from build123d import *

# Parameters (mm, degrees)
BOSS_EXTRUDE10_DEPTH = 2
SKETCH14_R           = 3
SKETCH14_R_2         = 5.05
BOSS_EXTRUDE11_DEPTH = 8


with BuildPart() as part:
    # Sketch13 → Boss-Extrude10 (new body)
    with BuildSketch(Plane(origin=(-28.225984218, 0, 0), x_dir=(-1, 0, 0), z_dir=(0, -1, 0))):
        with BuildLine():
            Line((-40.725984218, 11), (-15.725984218, 11))
            ThreePointArc((-15.725984218, 11), (-4.725984218, 0), (-15.725984218, -11))
            Line((-15.725984218, -11), (-40.725984218, -11))
            ThreePointArc((-40.725984218, -11), (-51.725984218, 0), (-40.725984218, 11))
        make_face()
    extrude(amount=BOSS_EXTRUDE10_DEPTH)

    # Sketch14 → Boss-Extrude11 (add)
    with BuildSketch(Plane.XZ):
        with Locations(Location((-11.5, 0, 0), (0, 0, 270))):
            Circle(SKETCH14_R)
        with Locations(Location((0, 0, 0), (0, 0, 270))):
            Circle(SKETCH14_R_2)
        with Locations(Location((11.5, 0, 0), (0, 0, 270))):
            Circle(SKETCH14_R)
    extrude(amount=-BOSS_EXTRUDE11_DEPTH)


solid = part.part
For this review, take the finished solid that the model builds, in its own axes (mm). A direction names the side the tool comes from. Give positions to 0.01 mm unless a question says otherwise; leave off trailing zeros. Loops run counter-clockwise (first coordinate to the right, second up) from the corner with the lowest first, then second, coordinate; pieces in that order, holes last. Notation, with made-up numbers: (15.25, 15) -> (64.25, 15) arc R13 ccw to (64.25, 36) -> close; hole circle Ø8 at (14, 55.5). An arc over 180 degrees is marked (long way). One line per question, with ' | ' between items.
1) We need section C-C (z = 0). Write out the cut boundary in (x, y).
Resolved:
outline: (-23.5, -2) -> (23.5, -2) -> (23.5, 0) -> (14.5, 0) -> (14.5, 8) -> (8.5, 8) -> (8.5, 0) -> (5.05, 0) -> (5.05, 8) -> (-5.05, 8) -> (-5.05, 0) -> (-8.5, 0) -> (-8.5, 8) -> (-14.5, 8) -> (-14.5, 0) -> (-23.5, 0) -> close
2) We need section A-A (x = -11.5). Write out the cut boundary in (y, z), plus the area to 3 significant figures.
Resolved:
outline: (-2, -11) -> (0, -11) -> (0, -3) -> (8, -3) -> (8, 3) -> (0, 3) -> (0, 11) -> (-2, 11) -> close | area: 92.0 mm2
3) The part is to be moulded in two halves that separate along X. For faces 3 (the cylindrical face through (-23.5, -1, -0.2)), 4 (the cylindrical face through (8.838, 3.944, -1.384)), 5 (the flat face through (0, -2, 0)), 6 (the cylindrical face through (-14.162, 3.944, -1.384)), say which applies: +X half, -X half, draft (parallel to the pull), parting line (faces both ways), or undercut.
Resolved:
face 3: -X half | face 4: undercut | face 5: draft | face 6: undercut
4) We need section D-D (x = 0). Write out the cut boundary in (y, z), plus the area to 3 significant figures.
Resolved:
outline: (-2, -11) -> (0, -11) -> (0, -5.05) -> (8, -5.05) -> (8, 5.05) -> (0, 5.05) -> (0, 11) -> (-2, 11) -> close | area: 125 mm2
5) We need section B-B (y = 5.25). Write out the cut boundary in (x, z), plus the area to 3 significant figures.
Resolved:
outline: circle Ø6 at (-11.5, 0); circle Ø10.1 at (0, 0); circle Ø6 at (11.5, 0) | area: 137 mm2
6) To check wall thickness, follow probe 1 along X at (y, z) = (6.25, -1); probe 2 along Y at (x, z) = (-20.5, -4.25); probe 3 along X at (y, z) = (7, -2.5). State the ranges of each line that lie inside material, in increasing order.
Resolved:
probe 1: x = -14.33 to -8.67, -4.95 to 4.95, 8.67 to 14.33 | probe 2: y = -2 to 0 | probe 3: x = -13.16 to -9.84, -4.39 to 4.39, 9.84 to 13.16
7) Insertion check: pin 1 Ø12 at (x, z) = (-11, -8.5) entering from +Y; pin 2 Ø6 at (y, z) = (4, 3) entering from -X; pin 3 Ø2 at (x, z) = (13, -8.5) entering from +Y; pin 4 Ø4 at (y, z) = (-1, -6.5) entering from +X. Each pin has a flat end and moves straight along its axis. Give the tip position at first contact, or say it passes through.
Resolved:
pin 1: stops at y = 8 | pin 2: stops at x = -14.5 | pin 3: stops at y = 0 | pin 4: stops at x = 22.54
8) For faces 1 (the cylindrical face through (-3.07, 3.94, 4.01)), 2 (the flat face through (0, -1, -11)), list the 3-axis set-ups (+Z, -Z, +X, -X, +Y, -Y) from which the entire face can be reached by the end or side of a thin tool; tool diameter is ignored.
Resolved:
face 1: +Y | face 2: -Z, +X, -X, +Y, -Y
